Input: part model. Units: mm. Frame: model coordinates. Face numbers are marked on the shaded views. Coordinates: 2 decimals unless noted, no trailing zeros. Write each loop counter-clockwise with the first axis right and the second up, starting at its lowest first coordinate (ties: lowest second). Pieces come first, ordered by that corner, then holes. Notation, with made-up numbers: (11.25, -10.75) - (59.25, -10.75) arc R21 ccw to (59.25, 28.25) - close; hole circle Ø9 at (25.5, 31.25). An arc over 180 degrees is marked (long way). Use CSV: the item, a comma, the result in double quotes.
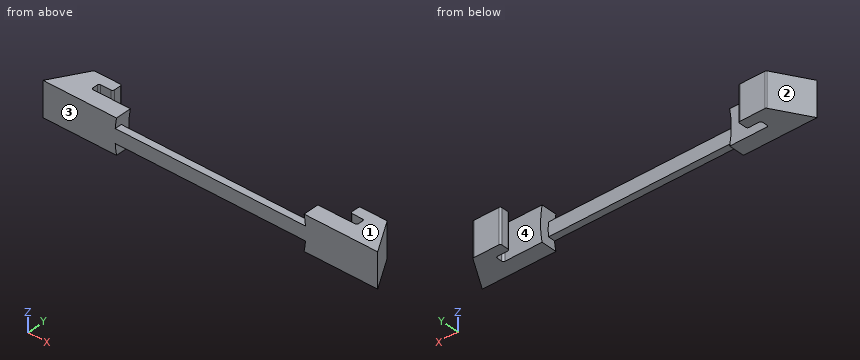
```python
from build123d import *

# Parameters (mm, degrees)
BOSS_EXTRUDE1_DEPTH     = 180
SKETCH2_W               = 91.04
SKETCH2_H               = 5.45
CUT_EXTRUDE1_DEPTH      = 30
SKETCH3_W               = 91.04
SKETCH3_H               = 5.45
CUT_EXTRUDE2_DEPTH      = 30
FILLET1_R               = 1
FILLET2_R               = 1
FILLET3_R               = 1
CUT_EXTRUDE3_DEPTH      = 200.714859237
CUT_EXTRUDE3_DEPTH_BACK = 200.714859237
SKETCH4_R               = 4
SKETCH4_R_2             = 27.5
CUT_EXTRUDE4_DEPTH      = 200.890776426
CUT_EXTRUDE4_DEPTH_BACK = 200.890776426
SKETCH6_W               = 96.5
SKETCH6_H               = 85
SKETCH7_W               = 55
SKETCH7_H               = 4
BOSS_EXTRUDE3_DEPTH     = 2


with BuildPart() as part:
    # Sketch1 → Boss-Extrude1 (new body)
    with BuildSketch(Plane.XY):
        with BuildLine():
            Line((-76.35, 0.5), (-76.35, 1.95))
            ThreePointArc((-76.35, 1.95), (-76.203553391, 2.303553391), (-75.85, 2.45))
            Line((-75.85, 2.45), (-72.85, 2.45))
            ThreePointArc((-72.85, 2.45), (-72.496446609, 2.596446609), (-72.35, 2.95))
            Line((-72.35, 2.95), (-72.35, 4.95))
            ThreePointArc((-72.35, 4.95), (-72.496446609, 5.303553391), (-72.85, 5.45))
            Line((-72.85, 5.45), (-79.85, 5.45))
            Line((-79.85, 5.45), (-80.066904811, 5.45))
            ThreePointArc((-80.066904811, 5.45), (-80.313254218, 5.385099953), (-80.495651273, 5.207247878))
            Line((-80.495651273, 5.207247878), (-86.35, -4.55))
            Line((-86.35, -4.55), (-80.35, -4.55))
            Line((-80.35, -4.55), (-79.85, -4.55))
            Line((-79.85, -4.55), (-38.1, -4.55))
            Line((-38.1, -4.55), (-38.1, 0))
            Line((-38.1, 0), (-75.85, 0))
            ThreePointArc((-75.85, 0), (-76.203553391, 0.146446609), (-76.35, 0.5))
        make_face()
        with BuildLine():
            Line((-0.35, 0), (-38.1, 0))
            Line((-38.1, 0), (-38.1, -4.55))
            Line((-38.1, -4.55), (3.65, -4.55))
            Line((3.65, -4.55), (4.15, -4.55))
            Line((4.15, -4.55), (10.15, -4.55))
            Line((10.15, -4.55), (4.295651273, 5.207247878))
            ThreePointArc((4.295651273, 5.207247878), (4.113254218, 5.385099953), (3.866904811, 5.45))
            Line((3.866904811, 5.45), (3.65, 5.45))
            Line((3.65, 5.45), (-3.35, 5.45))
            ThreePointArc((-3.35, 5.45), (-3.703553391, 5.303553391), (-3.85, 4.95))
            Line((-3.85, 4.95), (-3.85, 2.95))
            ThreePointArc((-3.85, 2.95), (-3.703553391, 2.596446609), (-3.35, 2.45))
            Line((-3.35, 2.45), (-0.35, 2.45))
            ThreePointArc((-0.35, 2.45), (0.003553391, 2.303553391), (0.15, 1.95))
            Line((0.15, 1.95), (0.15, 0.5))
            ThreePointArc((0.15, 0.5), (0.003553391, 0.146446609), (-0.35, 0))
        make_face()
    extrude(amount=BOSS_EXTRUDE1_DEPTH)

    # Sketch2 → Cut-Extrude1 (cut)
    with BuildSketch(Plane.XY.offset(180)):
        with Locations((-38.1, 2.725)):
            Rectangle(SKETCH2_W, SKETCH2_H)
    extrude(amount=-CUT_EXTRUDE1_DEPTH, mode=Mode.SUBTRACT)

    # Sketch3 → Cut-Extrude2 (cut)
    with BuildSketch(Plane(origin=(0, 0, 0), x_dir=(-1, 0, 0), z_dir=(0, 0, -1))):
        with Locations((38.1, 2.725)):
            Rectangle(SKETCH3_W, SKETCH3_H)
    extrude(amount=-CUT_EXTRUDE2_DEPTH, mode=Mode.SUBTRACT)

    # Fillet1
    fillet1_edges = [part.edges().sort_by_distance(p)[0] for p in [
        (-79.735, 0, 150),
    ]]
    fillet(fillet1_edges, radius=FILLET1_R)

    # Fillet2
    fillet2_edges = [part.edges().sort_by_distance(p)[0] for p in [
        (3.535, 0, 150),
    ]]
    fillet(fillet2_edges, radius=FILLET2_R)

    # Fillet3
    fillet3_edges = [part.edges().sort_by_distance(p)[0] for p in [
        (-79.735, 0, 30),
        (3.535, 0, 30),
    ]]
    fillet(fillet3_edges, radius=FILLET3_R)

    # Sketch4 → Cut-Extrude3 (cut, two sides: drawn at the far end of the back side and taken through both)
    with BuildSketch(Plane(origin=(0, 0, 0), x_dir=(1, 0, 0), z_dir=(0, 1, 0)).offset(-CUT_EXTRUDE3_DEPTH_BACK)):
        with BuildLine():
            Line((-28.1, -38), (-28.1, -2))
            ThreePointArc((-28.1, -2), (-27.514213562, -0.585786438), (-26.1, 0))
            Line((-26.1, 0), (-50.1, 0))
            ThreePointArc((-50.1, 0), (-48.685786438, -0.585786438), (-48.1, -2))
            Line((-48.1, -2), (-48.1, -38))
            ThreePointArc((-48.1, -38), (-47.514213562, -39.414213562), (-46.1, -40))
            Line((-46.1, -40), (-30.1, -40))
            ThreePointArc((-30.1, -40), (-28.685786438, -39.414213562), (-28.1, -38))
        make_face()
        with Locations(Location((-75.35, -10, 0), (0, 0, 270))):
            Circle(SKETCH4_R)
        with Locations(Location((-61.35, -20, 0), (0, 0, 270))):
            Circle(SKETCH4_R)
        with Locations(Location((-14.85, -20, 0), (0, 0, 270))):
            Circle(SKETCH4_R)
        with Locations(Location((-0.85, -10, 0), (0, 0, 270))):
            Circle(SKETCH4_R)
        with Locations(Location((-38.1, -90, 0), (0, 0, 270))):
            Circle(SKETCH4_R_2)
        with BuildLine():
            ThreePointArc((-30.1, -140), (-28.685786438, -140.585786438), (-28.1, -142))
            Line((-28.1, -142), (-28.1, -178))
            ThreePointArc((-28.1, -178), (-27.514213562, -179.414213562), (-26.1, -180))
            Line((-26.1, -180), (-50.1, -180))
            ThreePointArc((-50.1, -180), (-48.685786438, -179.414213562), (-48.1, -178))
            Line((-48.1, -178), (-48.1, -142))
            ThreePointArc((-48.1, -142), (-47.514213562, -140.585786438), (-46.1, -140))
            Line((-46.1, -140), (-30.1, -140))
        make_face()
        with Locations(Location((-61.35, -160, 0), (0, 0, 270))):
            Circle(SKETCH4_R)
        with Locations(Location((-75.35, -170, 0), (0, 0, 270))):
            Circle(SKETCH4_R)
        with Locations(Location((-14.85, -160, 0), (0, 0, 270))):
            Circle(SKETCH4_R)
        with Locations(Location((-0.85, -170, 0), (0, 0, 270))):
            Circle(SKETCH4_R)
    extrude(amount=CUT_EXTRUDE3_DEPTH + CUT_EXTRUDE3_DEPTH_BACK, mode=Mode.SUBTRACT)

    # Sketch6 → Cut-Extrude4 (cut, two sides: drawn at the far end of the back side and taken through both)
    with BuildSketch(Plane(origin=(0, 5.45, 0), x_dir=(1, 0, 0), z_dir=(0, 1, 0)).offset(-CUT_EXTRUDE4_DEPTH_BACK)):
        with Locations((-38.1, -137.5)):
            Rectangle(SKETCH6_W, SKETCH6_H)
        with Locations((-38.1, -42.5)):
            Rectangle(SKETCH6_W, SKETCH6_H)
    extrude(amount=CUT_EXTRUDE4_DEPTH + CUT_EXTRUDE4_DEPTH_BACK, mode=Mode.SUBTRACT)


with BuildPart() as cut_extrude4_piece_1:
    # of the separate pieces the step leaves, piece 1, a body of its own (cut_extrude4_pieces)
    add(part.part.solids().sort_by_distance((-0.35, 0, 85))[0])



with BuildPart() as cut_extrude4_piece_2:
    # of the separate pieces the step leaves, piece 2, a body of its own (cut_extrude4_pieces)
    add(part.part.solids().sort_by_distance((-65.141634566, 0, 85))[0])


with BuildPart() as cut_extrude4_piece_1_1:
    add(cut_extrude4_piece_1.part)

    add(cut_extrude4_piece_2.part)  # Boss-Extrude3 merges Cut-Extrude4 piece 2
    # Sketch7 → Boss-Extrude3 (add)
    with BuildSketch(Plane(origin=(0, -4.55, 0), x_dir=(1, 0, 0), z_dir=(0, 1, 0))):
        with Locations((-38.1, -89.999911505)):
            Rectangle(SKETCH7_W, SKETCH7_H)
    extrude(amount=BOSS_EXTRUDE3_DEPTH)


solid = cut_extrude4_piece_1_1.part
```
(1) Cut plane A-A on y = 4. Return loops of the section in (x, z), and give its area (3 significant figures).
Check values:
outline,"(-81.22, 85) - (-72.35, 85) - (-72.35, 95) - (-81.22, 95) - close; (-3.85, 85) - (5.02, 85) - (5.02, 95) - (-3.85, 95) - close"
area,"177 mm^2"
(2) Cut plane C-C on z = 90. Return loops of the section in (x, y), and give its area (3 significant figures).
Check values:
outline,"(-86.35, -4.55) - (10.15, -4.55) - (4.3, 5.21) arc R0.5 ccw to (3.87, 5.45) - (-3.35, 5.45) arc R0.5 ccw to (-3.85, 4.95) - (-3.85, 2.95) arc R0.5 ccw to (-3.35, 2.45) - (-0.35, 2.45) arc R0.5 cw to (0.15, 1.95) - (0.15, 0.5) arc R0.5 cw to (-0.35, 0) - (-10.6, 0) - (-10.6, -2.55) - (-65.6, -2.55) - (-65.6, 0) - (-75.85, 0) arc R0.5 cw to (-76.35, 0.5) - (-76.35, 1.95) arc R0.5 cw to (-75.85, 2.45) - (-72.85, 2.45) arc R0.5 ccw to (-72.35, 2.95) - (-72.35, 4.95) arc R0.5 ccw to (-72.85, 5.45) - (-80.07, 5.45) arc R0.5 ccw to (-80.5, 5.21) - close"
area,"372 mm^2"
(3) Ray query, probe 1 along Y at (x, z) = (-1.5, 85.5); probe 2 along X at (y, z) = (4.75, 88.5); probe 3 along X at (y, z) = (-0.25, 90.25). Return the intervals inside material, ascending. Write a range as from..to.
Check values:
probe 1,"-4.55..0, 2.45..5.45"
probe 2,"-80.77..-72.35, -3.85..4.57"
probe 3,"-83.77..-65.6, -10.6..7.57"
(4) Cut plane D-D on x = -68. Return loops of the section in (y, z).
Check values:
outline,"(-4.55, 85) - (0, 85) - (0, 95) - (-4.55, 95) - close"
(5) Cut plane B-B on y = -1.5. Return loops of the section in (x, z).
Check values:
outline,"(-84.52, 85) - (-65.14, 85) arc R27.5 cw to (-65.14, 95) - (-84.52, 95) - close; (-11.06, 85) - (8.32, 85) - (8.32, 95) - (-11.06, 95) arc R27.5 cw to start"
(6) Draft query along Y for the marked faces 1, 2, 3 and 4. Return one class per face: pulls with the +Y half, pulls with the -Y half, needs draft (parallel to the pull), parting line crosses it, or undercut.
Check values:
face 1,"needs draft"
face 2,"pulls with the +Y half"
face 3,"pulls with the -Y half"
face 4,"undercut"
(7) Pin query (flat end, axial travel): pin 1 Ø3 at (x, z) = (-9, 93) entering from +Y; pin 2 Ø2 at (x, y) = (-31, -3.5) entering from -Z; pin 3 Ø2 at (x, y) = (-38.5, -4) entering from +Z. Return the tip coordinate at first contact, or that it passes through.
Check values:
pin 1,"y = 0"
pin 2,"z = 88"
pin 3,"z = 92"
